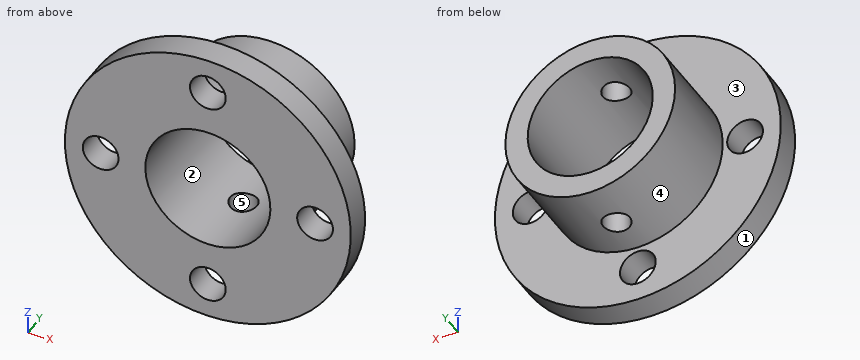
```python
from build123d import *

# Parameters (mm, degrees)
CUT_EXTRUDE1_DEPTH      = 27.095976701
CUT_EXTRUDE1_DEPTH_BACK = 27.095976701
SKETCH2_R               = 1.5
SKETCH3_R               = 2
CUT_EXTRUDE2_DEPTH      = 25.738633794
CIRPATTERN1_COUNT       = 4


with BuildPart() as part:
    # Sketch1 → Revolve1 (revolve)
    with BuildSketch(Plane(origin=(0, 0, 0), x_dir=(0, 0, -1), z_dir=(1, 0, 0)), mode=Mode.PRIVATE) as revolve1_sk:
        Polygon((-7, 0), (-16, 0), (-16, 3), (-9.5, 3), (-9.5, 13), (-7, 13), align=None)
    revolve(revolve1_sk.sketch.rotate(Axis((0, 0, 0), (0, 1, 0)), 180), axis=Axis((0, 0, 0), (0, 1, 0)))

    # Sketch2 → Cut-Extrude1 (cut, two sides: drawn at the far end of the back side and taken through both)
    with BuildSketch(Plane.XY.offset(-CUT_EXTRUDE1_DEPTH_BACK)):
        with Locations((0, 7.5)):
            Circle(SKETCH2_R)
    extrude(amount=CUT_EXTRUDE1_DEPTH + CUT_EXTRUDE1_DEPTH_BACK, mode=Mode.SUBTRACT)

    # Sketch3 → Cut-Extrude2 (cut, symmetric)
    with BuildSketch(Plane(origin=(0, 3, 0), x_dir=(1, 0, 0), z_dir=(0, 1, 0))):
        with Locations(Location((0, -12, 0), (0, 0, 270))):
            Circle(SKETCH3_R)
    cut_extrude2 = extrude(amount=CUT_EXTRUDE2_DEPTH, both=True, mode=Mode.SUBTRACT)

    # CirPattern1: Cut-Extrude2 ×4 about axis
    cirpattern1_axis = Axis((0, 0, 0), (0, 1, 0))
    for i in range(1, CIRPATTERN1_COUNT):
        add(cut_extrude2.rotate(cirpattern1_axis, i * 360 / CIRPATTERN1_COUNT), mode=Mode.SUBTRACT)


solid = part.part
```
Can you work these out from the model? Positions are in its coordinate system, mm. Face numbers are marked on the shaded views. A direction names the side the tool comes from. Give positions to 0.01 mm unless a question says otherwise; leave off trailing zeros. Order: outer loops, then holes, each group sorted by start corner. A loop starts at its lowest first (then second) coordinate and runs counter-clockwise, first axis right, second up. Notation, with made-up numbers: (40, 2.5) - (83, 2.5) arc R28 ccw to (83, 41.5) - close; hole circle Ø1 at (61, -21.75). An arc over 180 degrees is marked (long way). Use a Markdown table: item, result. Add a question column.
Q1. If we section it at B-B on z = 0: Write out the boundary of the cut face in (x, y).
Q2. If we mould it in two halves opening along Z, with no side actions, what happens to the marked faces 1, 2 and 3? For each: released by +Z, released by -Z, zero draft, split by the parting line, or undercut.
Q3. I'm going to push flat-ended pins straight in: pin 1 (4 mm diameter, centred on x = -10.5, y = 3, fed in from +Z); pin 2 (6 mm diameter, centred on x = -10, y = 2, fed in from -Z); pin 3 (3 mm diameter, centred on x = 8, y = 2, fed in from +Z). Where does each tip first touch, or does it pass through?
Q4. On a 3-axis mill with a long thin cutter (end or side, diameter ignored), from which of +Z, -Z, +X, -X, +Y, -Y can I reach the whole of each face in a straight line? I mean the marked faces 4 and 5. Say none if no direction works.
Q5. If we section it at D-D on z = 12: Write out the boundary of the cut face in (x, y), plus the area to 3 significant figures.
Q6. If we section it at C-C on y = 7.5: Write out the boundary of the cut face in (x, z).
Q7. If we section it at A-A on x = 0: Write out the boundary of the cut face in (y, z).
Q8. Please list where these lines run through material, in increasing order: line 1 along X through (y, z) = (4.75, 2); line 2 along Y through (x, z) = (6, -10.5); line 3 along X through (y, z) = (7.5, 7.8).
Answers follow:
| question | item | result |
|---|---|---|
| 1 | outline | (-16, 0) - (-14, 0) - (-14, 3) - (-16, 3) - close; (-10, 0) - (-7, 0) - (-7, 13) - (-9.5, 13) - (-9.5, 3) - (-10, 3) - close; (7, 0) - (10, 0) - (10, 3) - (9.5, 3) - (9.5, 13) - (7, 13) - close; (14, 0) - (16, 0) - (16, 3) - (14, 3) - close |
| 2 | face 1 | split by the parting line |
| 2 | face 2 | undercut |
| 2 | face 3 | zero draft |
| 3 | pin 1 | stops at z = 13.56 |
| 3 | pin 2 | stops at z = -14.39 |
| 3 | pin 3 | stops at z = 14.62 |
| 4 | face 4 | +Y |
| 4 | face 5 | +Z, -Z |
| 5 | outline | (-10.58, 0) - (-2, 0) - (-2, 3) - (-10.58, 3) - close; (2, 0) - (10.58, 0) - (10.58, 3) - (2, 3) - close |
| 5 | area | 51.5 mm^2 |
| 6 | outline | (-1.5, -9.38) - (-1.5, -6.84) arc R7 cw to (-1.5, 6.84) - (-1.5, 9.38) arc R9.5 ccw to start; (1.5, -9.38) arc R9.5 ccw to (1.5, 9.38) - (1.5, 6.84) arc R7 cw to (1.5, -6.84) - close |
| 7 | outline | (0, -16) - (3, -16) - (3, -14) - (0, -14) - close; (0, -10) - (3, -10) - (3, -9.5) - (6, -9.5) - (6, -7) - (0, -7) - close; (0, 7) - (6, 7) - (6, 9.5) - (3, 9.5) - (3, 10) - (0, 10) - close; (0, 14) - (3, 14) - (3, 16) - (0, 16) - close; (9, -9.5) - (13, -9.5) - (13, -7) - (9, -7) - close; (9, 7) - (13, 7) - (13, 9.5) - (9, 9.5) - close |
| 8 | line 1 | x = -9.29 to -6.71, 6.71 to 9.29 |
| 8 | line 2 | y = 0 to 3 |
| 8 | line 3 | x = -5.42 to -1.5, 1.5 to 5.42 |
